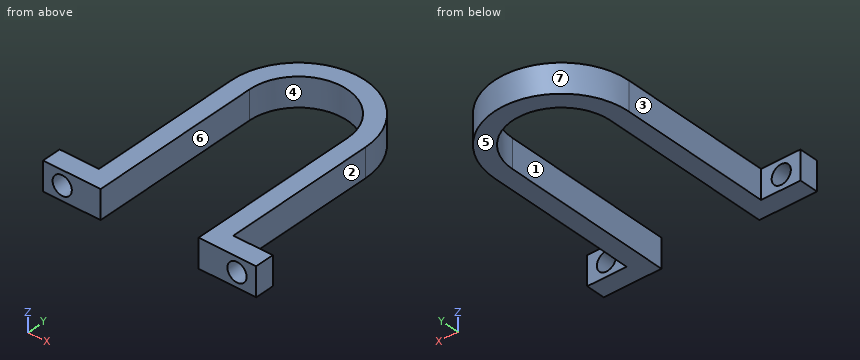
```python
from build123d import *

# Parameters (mm, degrees)
BOSS_EXTRUDE1_DEPTH = 15
SKETCH3_R           = 5
CUT_EXTRUDE2_DEPTH  = 138.587245048


with BuildPart() as part:
    # Sketch1 → Boss-Extrude1 (new body)
    with BuildSketch(Plane.XY):
        with BuildLine():
            Line((55.5, -90), (55.5, -80))
            Line((55.5, -80), (35, -80))
            Line((35, -80), (35, 0))
            ThreePointArc((35, 0), (0, 35), (-35, 0))
            Line((-35, 0), (-35, -80))
            Line((-35, -80), (-55.5, -80))
            Line((-55.5, -80), (-55.5, -90))
            Line((-55.5, -90), (-25.5, -90))
            Line((-25.5, -90), (-25.5, 0))
            ThreePointArc((-25.5, 0), (0, 25.5), (25.5, 0))
            Line((25.5, 0), (25.5, -90))
            Line((25.5, -90), (55.5, -90))
        make_face()
    extrude(amount=BOSS_EXTRUDE1_DEPTH)

    # Sketch3 → Cut-Extrude2 (cut, through all)
    with BuildSketch(Plane.XZ.offset(90)):
        with Locations(Location((-45.5, 7.5, 0), (0, 0, 270))):
            Circle(SKETCH3_R)
        with Locations(Location((45.5, 7.5, 0), (0, 0, 270))):
            Circle(SKETCH3_R)
    extrude(amount=-CUT_EXTRUDE2_DEPTH, mode=Mode.SUBTRACT)


solid = part.part
```
Part model, mm, in its own coordinate system. Face numbers are marked on the shaded views. A direction names the side the tool comes from. Give positions to 0.01 mm unless a question says otherwise; leave off trailing zeros. Write each loop counter-clockwise with the first axis right and the second up, starting at its lowest first coordinate (ties: lowest second). Pieces come first, ordered by that corner, then holes. Notation, with made-up numbers: (40.25, 44) -> (64.25, 44) arc R3 ccw to (64.25, 49) -> close; hole circle Ø3 at (45.5, 81.25). An arc over 180 degrees is marked (long way). Put each result on its own line as item: value. Start each with the question number.
Item 1: Pull direction X, two halves, no side cores. Call the marked faces 4, 5, 6 and 7: pulls with the +X half, pulls with the -X half, needs draft (parallel to the pull), parting line crosses it, or undercut.
Item 2: Pin check, flat tips, straight feed: pin 1 Ø4.5 at (y, z) = (-50.5, 10) entering from -X; pin 2 Ø4.5 at (x, z) = (-40.5, 10.5) entering from +Y; pin 3 Ø1.5 at (x, z) = (-13, 8.5) entering from +Y. Stop position of each tip, or through.
Item 3: Which spindle directions (+Z, -Z, +X, -X, +Y, -Y) get a long thin tool onto all of the face, cutting with end or side? Do the marked faces 1, 2 and 3. Say none if no direction does.
Item 4: Cut at B-B (z = 7.5). List the corners of the cut face in (x, y), then the cut area to 3 significant figures.
Item 5: Cut at A-A (y = -64). List the corners of the cut face in (x, z), then the cut area to 3 significant figures.
Item 6: Cut at C-C (x = 45.5). List the corners of the cut face in (y, z), then the cut area to 3 significant figures.
Item 7: Cut at D-D (x = 0). List the corners of the cut face in (y, z).
Item 8: Wall check: L1, parallel to X at y = -87.5, z = 7.5; L2, parallel to X at y = -9, z = 14.25; L3, parallel to Y at x = -42, z = 3.25. Give the ranges that are in metal, low to high. Write a range as [from, to].
Answer list:
1. face 4: undercut
1. face 5: needs draft
1. face 6: undercut
1. face 7: parting line crosses it
2. pin 1: stops at x = -35
2. pin 2: stops at y = -80
2. pin 3: stops at y = 32.79
3. face 1: +Z, -Z, -Y
3. face 2: +Z, -Z, +X, +Y
3. face 3: +Z, -Z, -X, +Y
4. outline: (-55.5, -90) -> (-50.5, -90) -> (-50.5, -80) -> (-55.5, -80) -> close; (-40.5, -90) -> (-25.5, -90) -> (-25.5, 0) arc R25.5 cw to (25.5, 0) -> (25.5, -90) -> (40.5, -90) -> (40.5, -80) -> (35, -80) -> (35, 0) arc R35 ccw to (-35, 0) -> (-35, -80) -> (-40.5, -80) -> close; (50.5, -90) -> (55.5, -90) -> (55.5, -80) -> (50.5, -80) -> close
4. area: 2,820 mm2
5. outline: (-35, 0) -> (-25.5, 0) -> (-25.5, 15) -> (-35, 15) -> close; (25.5, 0) -> (35, 0) -> (35, 15) -> (25.5, 15) -> close
5. area: 285 mm2
6. outline: (-90, 0) -> (-80, 0) -> (-80, 2.5) -> (-90, 2.5) -> close; (-90, 12.5) -> (-80, 12.5) -> (-80, 15) -> (-90, 15) -> close
6. area: 50.0 mm2
7. outline: (25.5, 0) -> (35, 0) -> (35, 15) -> (25.5, 15) -> close
8. L1: x = [-55.5, -50.5], [-40.5, -25.5], [25.5, 40.5], [50.5, 55.5]
8. L2: x = [-35, -25.5], [25.5, 35]
8. L3: y = [-90, -80]
